For this review, take the finished solid that the model builds, in its own axes (mm). Give positions to 0.01 mm unless a question says otherwise; leave off trailing zeros. Loops run counter-clockwise (first coordinate to the right, second up) from the corner with the lowest first, then second, coordinate; pieces in that order, holes last. Notation, with made-up numbers: (4.5, -25.75) - (43.5, -25.75) arc R15 ccw to (43.5, 3.25) - close; hole circle Ø6 at (-39.75, 80.25). An arc over 180 degrees is marked (long way). Put each result on its own line as item: value. Start each with the question number.
from build123d import *

# Parameters (mm, degrees)
SKETCH_1_W          = 5
SKETCH_1_H          = 30
EXTRUDE_1_DEPTH     = 130
SKETCH_2_R          = 22.5
EXTRUDE_2_DEPTH     = 5
SKETCH_3_R          = 13
CUT_EXTRUDE_1_DEPTH = 136.392946641
HOLE_WIZARD_M33_D   = 3.4
HOLE_WIZARD_M32_D   = 3.4
EXTRUDE_3_DEPTH     = 5
HOLE_WIZARD_M31_D   = 3.4
SKETCH_14_W         = 45
SKETCH_14_H         = 6
CUT_EXTRUDE_2_DEPTH = 1
CUT_EXTRUDE_3_REACH = 137.393
FILLET_1_R          = 2
FILLET_2_R          = 2


with BuildPart() as part:
    # Эскиз1 → Бобышка-Вытянуть1 (new body)
    with BuildSketch(Plane(origin=(0, 0, 0), x_dir=(1, 0, 0), z_dir=(0, 1, 0))):
        with Locations((2.5, -15)):
            Rectangle(SKETCH_1_W, SKETCH_1_H)
    extrude(amount=EXTRUDE_1_DEPTH)

    # Эскиз2 → Бобышка-Вытянуть2 (add)
    with BuildSketch(Plane.ZY):
        with Locations((15, 65)):
            Circle(SKETCH_2_R)
    extrude(amount=-EXTRUDE_2_DEPTH)

    # Эскиз3 → Вырез-Вытянуть1 (cut, through all)
    with BuildSketch(Plane.ZY):
        with Locations((15, 65)):
            Circle(SKETCH_3_R)
    extrude(amount=-CUT_EXTRUDE_1_DEPTH, mode=Mode.SUBTRACT)

    # Отверстие с зазором M33 (through all)
    with Locations(Plane(origin=(5, -25.024735225, 7.262908886), x_dir=(0, 0, 1), z_dir=(1, 0, 0))):
        with Locations((7.737091114, -109.274735225), (-11.512908886, -90.024735225), (7.737091114, -70.774735225), (26.987091114, -90.024735225)):
            Hole(HOLE_WIZARD_M33_D / 2)

    # Отверстие с зазором M32 (through all)
    with Locations(Plane(origin=(5, 0, 0), x_dir=(0, 0, -1), z_dir=(1, 0, 0))):
        with Locations((-26, 106), (-4, 106), (-4, 24), (-26, 24)):
            Hole(HOLE_WIZARD_M32_D / 2)

    # Эскиз11 → Бобышка-Вытянуть3 (add)
    with BuildSketch(Plane(origin=(5, 0, 0), x_dir=(0, 0, -1), z_dir=(1, 0, 0))):
        Polygon((-37.5, 124), (-30, 111.009618943), (0, 111.009618943), (7.5, 124), (7.5, 130), (-37.5, 130), align=None)
        Polygon((0, 18.990381057), (7.5, 6), (7.5, 0), (-37.5, 0), (-37.5, 6), (-30, 18.990381057), align=None)
    extrude(amount=-EXTRUDE_3_DEPTH)

    # Отверстие с зазором M31 (through all)
    with Locations(Plane(origin=(5, 0, 0), x_dir=(0, 0, -1), z_dir=(1, 0, 0))):
        with Locations((-28.5, 127), (-19.5, 127), (-10.5, 127), (-1.5, 127), (-28.5, 3), (-19.5, 3), (-10.5, 3), (-1.5, 3)):
            Hole(HOLE_WIZARD_M31_D / 2)

    # Эскиз14 → Вырез-Вытянуть2 (cut)
    with BuildSketch(Plane(origin=(5, 0, 0), x_dir=(0, 0, -1), z_dir=(1, 0, 0))):
        with Locations((-15, 127)):
            Rectangle(SKETCH_14_W, SKETCH_14_H)
        with Locations((-15, 3)):
            Rectangle(SKETCH_14_W, SKETCH_14_H)
    extrude(amount=-CUT_EXTRUDE_2_DEPTH, mode=Mode.SUBTRACT)

    # Эскиз15 → Вырез-Вытянуть3 (cut, up to next)
    with BuildSketch(Plane(origin=(5, 0, 0), x_dir=(0, 0, -1), z_dir=(1, 0, 0)), mode=Mode.PRIVATE) as cut_extrude_3_sk1:
        with BuildLine():
            Line((-17, 42.589065169), (-17, 36.505828051))
            Line((-17, 36.505828051), (-26, 33.230095943))
            Line((-26, 33.230095943), (-26, 45.372213574))
            ThreePointArc((-26, 45.372213574), (-21.647291084, 43.504337153), (-17, 42.589065169))
        make_face()
    cut_extrude_3_tool1 = extrude(cut_extrude_3_sk1.sketch, amount=-CUT_EXTRUDE_3_REACH, mode=Mode.PRIVATE) & part.part
    # Эскиз15 → Вырез-Вытянуть3 (cut, up to next)
    with BuildSketch(Plane(origin=(5, 0, 0), x_dir=(0, 0, -1), z_dir=(1, 0, 0)), mode=Mode.PRIVATE) as cut_extrude_3_sk2:
        with BuildLine():
            Line((-13, 42.589065169), (-13, 36.505828051))
            Line((-13, 36.505828051), (-4, 33.230095943))
            Line((-4, 33.230095943), (-4, 45.372213574))
            ThreePointArc((-4, 45.372213574), (-8.352708916, 43.504337153), (-13, 42.589065169))
        make_face()
    cut_extrude_3_tool2 = extrude(cut_extrude_3_sk2.sketch, amount=-CUT_EXTRUDE_3_REACH, mode=Mode.PRIVATE) & part.part
    # Эскиз15 → Вырез-Вытянуть3 (cut, up to next)
    with BuildSketch(Plane(origin=(5, 0, 0), x_dir=(0, 0, -1), z_dir=(1, 0, 0)), mode=Mode.PRIVATE) as cut_extrude_3_sk3:
        Polygon((-15, 32.97705743), (-22.461792276, 30.261187147), (-15, 24), (-7.538207724, 30.261187147), align=None)
    cut_extrude_3_tool3 = extrude(cut_extrude_3_sk3.sketch, amount=-CUT_EXTRUDE_3_REACH, mode=Mode.PRIVATE) & part.part
    # Эскиз15 → Вырез-Вытянуть3 (cut, up to next)
    with BuildSketch(Plane(origin=(5, 0, 0), x_dir=(0, 0, -1), z_dir=(1, 0, 0)), mode=Mode.PRIVATE) as cut_extrude_3_sk4:
        Polygon((-15, 23.9), (-26, 14.669904057), (-26, 10), (-4, 10), (-4, 14.669904057), align=None)
    cut_extrude_3_tool4 = extrude(cut_extrude_3_sk4.sketch, amount=-CUT_EXTRUDE_3_REACH, mode=Mode.PRIVATE) & part.part
    # Эскиз15 → Вырез-Вытянуть3 (cut, up to next)
    with BuildSketch(Plane(origin=(5, 0, 0), x_dir=(0, 0, -1), z_dir=(1, 0, 0)), mode=Mode.PRIVATE) as cut_extrude_3_sk5:
        with BuildLine():
            Line((-13, 87.410934831), (-13, 93.494171949))
            Line((-13, 93.494171949), (-4, 96.769904057))
            Line((-4, 96.769904057), (-4, 84.627786426))
            ThreePointArc((-4, 84.627786426), (-8.352708916, 86.495662847), (-13, 87.410934831))
        make_face()
    cut_extrude_3_tool5 = extrude(cut_extrude_3_sk5.sketch, amount=-CUT_EXTRUDE_3_REACH, mode=Mode.PRIVATE) & part.part
    # Эскиз15 → Вырез-Вытянуть3 (cut, up to next)
    with BuildSketch(Plane(origin=(5, 0, 0), x_dir=(0, 0, -1), z_dir=(1, 0, 0)), mode=Mode.PRIVATE) as cut_extrude_3_sk6:
        with BuildLine():
            Line((-26, 96.769904057), (-26, 84.627786426))
            ThreePointArc((-26, 84.627786426), (-21.647291084, 86.495662847), (-17, 87.410934831))
            Line((-17, 87.410934831), (-17, 93.494171949))
            Line((-17, 93.494171949), (-26, 96.769904057))
        make_face()
    cut_extrude_3_tool6 = extrude(cut_extrude_3_sk6.sketch, amount=-CUT_EXTRUDE_3_REACH, mode=Mode.PRIVATE) & part.part
    # Эскиз15 → Вырез-Вытянуть3 (cut, up to next)
    with BuildSketch(Plane(origin=(5, 0, 0), x_dir=(0, 0, -1), z_dir=(1, 0, 0)), mode=Mode.PRIVATE) as cut_extrude_3_sk7:
        Polygon((-7.538207724, 99.738812853), (-15, 97.02294257), (-22.461792276, 99.738812853), (-15, 106), align=None)
    cut_extrude_3_tool7 = extrude(cut_extrude_3_sk7.sketch, amount=-CUT_EXTRUDE_3_REACH, mode=Mode.PRIVATE) & part.part
    # Эскиз15 → Вырез-Вытянуть3 (cut, up to next)
    with BuildSketch(Plane(origin=(5, 0, 0), x_dir=(0, 0, -1), z_dir=(1, 0, 0)), mode=Mode.PRIVATE) as cut_extrude_3_sk8:
        Polygon((-4, 120), (-4, 115.330095943), (-15, 106.1), (-26, 115.330095943), (-26, 120), align=None)
    cut_extrude_3_tool8 = extrude(cut_extrude_3_sk8.sketch, amount=-CUT_EXTRUDE_3_REACH, mode=Mode.PRIVATE) & part.part
    add(cut_extrude_3_tool1.solids().sort_by_distance((5, 39.236423, 22.016157))[0], mode=Mode.SUBTRACT)
    add(cut_extrude_3_tool2.solids().sort_by_distance((5, 39.236423, 7.983843))[0], mode=Mode.SUBTRACT)
    add(cut_extrude_3_tool3.solids().sort_by_distance((5, 29.079415, 15))[0], mode=Mode.SUBTRACT)
    add(cut_extrude_3_tool4.solids().sort_by_distance((5, 15.024791, 15))[0], mode=Mode.SUBTRACT)
    add(cut_extrude_3_tool5.solids().sort_by_distance((5, 90.763577, 7.983843))[0], mode=Mode.SUBTRACT)
    add(cut_extrude_3_tool6.solids().sort_by_distance((5, 90.763577, 22.016157))[0], mode=Mode.SUBTRACT)
    add(cut_extrude_3_tool7.solids().sort_by_distance((5, 100.920585, 15))[0], mode=Mode.SUBTRACT)
    add(cut_extrude_3_tool8.solids().sort_by_distance((5, 114.975209, 15))[0], mode=Mode.SUBTRACT)

    # Скругление1
    fillet_1_edges = [part.edges().sort_by_distance(p)[0] for p in [
        (2.5, 18.990381057, 30),
        (2.5, 18.990381057, 0),
        (2.5, 48.229490169, 0),
        (2.5, 81.770509831, 0),
        (2.5, 48.229490169, 30),
        (2.5, 81.770509831, 30),
        (2.5, 111.009618943, 0),
        (2.5, 111.009618943, 30),
    ]]
    fillet(fillet_1_edges, radius=FILLET_1_R)

    # Скругление2
    fillet_2_edges = [part.edges().sort_by_distance(p)[0] for p in [
        (2.5, 45.372213574, 26),
        (2.5, 42.589065169, 17),
        (2.5, 33.230095943, 26),
        (2.5, 42.589065169, 13),
        (2.5, 45.372213574, 4),
        (2.5, 33.230095943, 4),
        (2.5, 36.505828051, 13),
        (2.5, 32.97705743, 15),
        (2.5, 30.261187147, 7.538207724),
        (2.5, 24, 15),
        (2.5, 30.261187147, 22.461792276),
        (2.5, 23.9, 15),
        (2.5, 14.669904057, 4),
        (2.5, 10, 4),
        (2.5, 10, 26),
        (2.5, 14.669904057, 26),
        (2.5, 84.627786426, 4),
        (2.5, 87.410934831, 13),
        (2.5, 93.494171949, 13),
        (2.5, 96.769904057, 4),
        (2.5, 87.410934831, 17),
        (2.5, 84.627786426, 26),
        (2.5, 96.769904057, 26),
        (2.5, 93.494171949, 17),
        (2.5, 106, 15),
        (2.5, 99.738812853, 7.538207724),
        (2.5, 97.02294257, 15),
        (2.5, 99.738812853, 22.461792276),
        (2.5, 120, 26),
        (2.5, 120, 4),
        (2.5, 115.330095943, 4),
        (2.5, 106.1, 15),
        (2.5, 115.330095943, 26),
    ]]
    fillet(fillet_2_edges, radius=FILLET_2_R)


solid = part.part
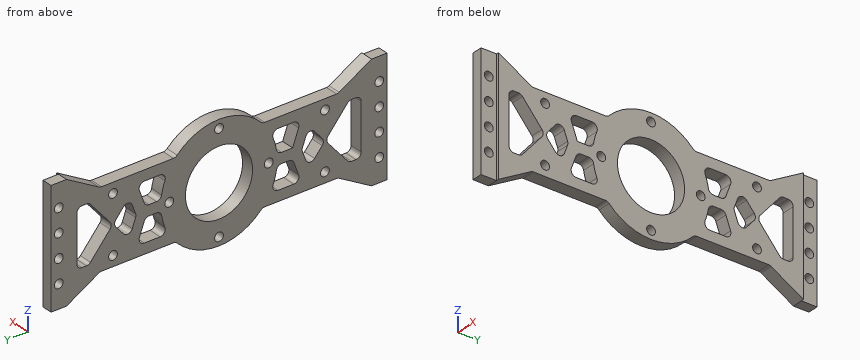
1) Take a section at A-A on y = 65. State the section outline as (x, z) points, and give its area (3 significant figures).
2) Take a section at B-B on y = 45.75. State the section outline as (x, z) points.
3) Wall thickness on probe 1 along Y at (x, z) = (2.5, 1.5); probe 2 along Y at (x, z) = (3.4, -4.25); probe 3 along Z at (x, y) = (0.7, 42.5): over which ranges is each line inside the solid? List them lowest first.
4) Insertion check: P1, Ø4.5, axis at y = 3, z = 19.5, coming from the +X side; P2, Ø3, axis at x = 1.5, y = 91, coming from the -Z side; P3, Ø0.8, axis at x = 4.5, z = 18.5, coming from the +Y side. Each pin has a flat end and moves straight along its axis. Give the tip position at first contact, or say it passes through.
5) Take a section at D-D on x = 1.7. State how many separate pieces and enclosed holes the cut face has, and give its area (3 significant figures).
6) Take a section at C-C on z = -4.25. State the section outline as (x, y) points, and give its area (3 significant figures).
Answers follow:
1. outline: (0, -7.5) - (5, -7.5) - (5, -5.95) - (0, -5.95) - close; (0, -2.55) - (5, -2.55) - (5, 2) - (0, 2) - close; (0, 28) - (5, 28) - (5, 32.55) - (0, 32.55) - close; (0, 35.95) - (5, 35.95) - (5, 37.5) - (0, 37.5) - close
1. area: 61.0 mm2
2. outline: (0, 0) - (5, 0) - (5, 13.3) - (0, 13.3) - close; (0, 16.7) - (5, 16.7) - (5, 30) - (0, 30) - close
3. probe 1: 0 to 1.3, 4.7 to 125.3, 128.7 to 130
3. probe 2: 0 to 11.63, 53.35 to 63.3, 66.7 to 76.65, 118.37 to 130
3. probe 3: 0 to 4.02, 12.1 to 17.9, 25.98 to 30
4. P1: x = 4
4. P2: z = 0
4. P3: y = 124
5. separate pieces: 1
5. enclosed holes: 25
5. area: 3,130 mm2
6. outline: (0, 0) - (4, 0) - (4, 6) - (5, 6) - (5, 11.63) - (0, 11.63) - close; (0, 53.35) - (5, 53.35) - (5, 63.3) - (0, 63.3) - close; (0, 66.7) - (5, 66.7) - (5, 76.65) - (0, 76.65) - close; (0, 118.37) - (5, 118.37) - (5, 124) - (4, 124) - (4, 130) - (0, 130) - close
6. area: 204 mm2
